```python
from build123d import *

# Parameters (mm, degrees)
SKETCH1_R           = 4.5
SKETCH1_R_2         = 4.15
SKETCH1_R_3         = 1.5
BOSS_EXTRUDE2_DEPTH = 4


with BuildPart() as part:
    # Sketch1 → Boss-Extrude2 (new body)
    with BuildSketch(Plane(origin=(0, 0, 0), x_dir=(1, 0, 0), z_dir=(0, 1, 0))):
        with BuildLine():
            Line((24.492030041, 32), (-16.82364897, 31.38929644))
            ThreePointArc((-16.82364897, 31.38929644), (-26.628373919, 32.520273369), (-35.798432863, 36.170171872))
            Line((-35.798432863, 36.170171872), (-38.479754021, 32.316380416))
            ThreePointArc((-38.479754021, 32.316380416), (-38.105147294, 30.228398184), (-40.193129525, 29.853791457))
            Line((-40.193129525, 29.853791457), (-42.874450683, 26))
            ThreePointArc((-42.874450683, 26), (-33.263093393, 21.189213431), (-22.681899906, 19.302363998))
            Line((-22.681899906, 19.302363998), (24.519122197, 20.000061166))
            ThreePointArc((24.519122197, 20.000061166), (29.912542793, 18.512398384), (34.38564897, 15.151825901))
            ThreePointArc((34.38564897, 15.151825901), (39.572200335, 12.78648108), (44.865586737, 14.901955396))
            ThreePointArc((44.865586737, 14.901955396), (46.941127439, 15.77786367), (49.041095181, 14.962253472))
            ThreePointArc((49.041095181, 14.962253472), (51.498094019, 13.563547988), (54.322847672, 13.445280812))
            ThreePointArc((54.322847672, 13.445280812), (60.067220976, 15.331144894), (65.190877045, 18.540888881))
            ThreePointArc((65.190877045, 18.540888881), (68.785066518, 26.1), (65.156781581, 33.642805002))
            ThreePointArc((65.156781581, 33.642805002), (60.018684596, 36.829381119), (54.265854499, 38.689288065))
            ThreePointArc((54.265854499, 38.689288065), (51.441663661, 38.558267317), (48.991005527, 37.148481859))
            ThreePointArc((48.991005527, 37.148481859), (46.894741967, 36.323397867), (44.815267383, 37.189925399))
            ThreePointArc((44.815267383, 37.189925399), (39.512382816, 39.281476607), (34.336564706, 36.892736755))
            ThreePointArc((34.336564706, 36.892736755), (29.878678322, 33.512000849), (24.492030041, 32))
        make_face()
        with Locations(Location((59.085066518, 26.078100395, 0), (0, 0, 270))):
            Circle(SKETCH1_R, mode=Mode.SUBTRACT)
        with Locations(Location((45.985066518, 26.04852464, 0), (0, 0, 270))):
            Circle(SKETCH1_R_2, mode=Mode.SUBTRACT)
        with Locations(Location((-20.570161775, 25.66516132, 0), (0, 0, 270))):
            Circle(SKETCH1_R_3, mode=Mode.SUBTRACT)
        with BuildLine():
            Line((39.841844345, 34.144341712), (40.83090249, 33.199674393))
            ThreePointArc((40.83090249, 33.199674393), (40.883202658, 30.92140707), (38.604935336, 30.869106902))
            Line((38.604935336, 30.869106902), (37.615877191, 31.813774221))
            ThreePointArc((37.615877191, 31.813774221), (37.563577023, 34.092041544), (39.841844345, 34.144341712))
        make_face(mode=Mode.SUBTRACT)
        with BuildLine():
            Line((52.091670541, 34.171998037), (51.106887992, 33.222874395))
            ThreePointArc((51.106887992, 33.222874395), (51.064875553, 30.944394144), (53.343355804, 30.902381704))
            Line((53.343355804, 30.902381704), (54.328138354, 31.851505346))
            ThreePointArc((54.328138354, 31.851505346), (54.370150793, 34.129985598), (52.091670541, 34.171998037))
        make_face(mode=Mode.SUBTRACT)
        with BuildLine():
            Line((52.128288691, 17.952707568), (51.139230546, 18.897374887))
            ThreePointArc((51.139230546, 18.897374887), (51.086930378, 21.17564221), (53.365197701, 21.227942378))
            Line((53.365197701, 21.227942378), (54.354255846, 20.283275059))
            ThreePointArc((54.354255846, 20.283275059), (54.406556014, 18.005007736), (52.128288691, 17.952707568))
        make_face(mode=Mode.SUBTRACT)
        with BuildLine():
            Line((39.878462495, 17.925051243), (40.863245045, 18.874174885))
            ThreePointArc((40.863245045, 18.874174885), (40.905257484, 21.152655136), (38.626777232, 21.194667576))
            Line((38.626777232, 21.194667576), (37.641994683, 20.245543933))
            ThreePointArc((37.641994683, 20.245543933), (37.599982244, 17.967063682), (39.878462495, 17.925051243))
        make_face(mode=Mode.SUBTRACT)
    extrude(amount=BOSS_EXTRUDE2_DEPTH)


solid = part.part
```
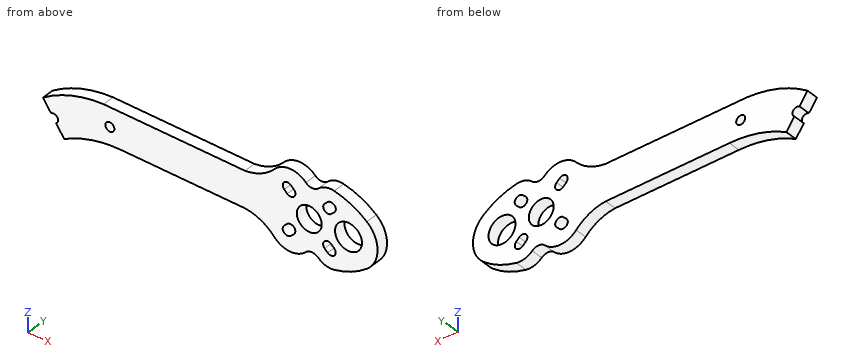
Verification items for the finished model (mm, model axes). Coordinates: 2 decimals unless noted, no trailing zeros. Loops run counter-clockwise (first coordinate to the right, second up) from the corner with the lowest first, then second, coordinate; pieces in that order, holes last. Notation, with made-up numbers: (8.25, 26) - (12.25, 26) arc R18 ccw to (12.25, 41) - close; hole circle Ø4 at (77, 24). An arc over 180 degrees is marked (long way). Put each result on its own line as item: value.
Item 1: Section check D-D (x = -24). Enter the section's corners in (y, z).
Conclusion:
outline: (0, -31.96) - (4, -31.96) - (4, -19.37) - (0, -19.37) - close
Item 2: Gauge pin test, flat end, axial feed: pin 1 Ø5 at (x, z) = (-20.57, -25.67) entering from -Y. Record the tip position at first contact, or that the pin passes through.
Conclusion:
pin 1: stops at y = 0
Item 3: Section check A-A (z = -23). Enter the section's corners in (x, y), then the cut area to 3 significant figures.
Conclusion:
outline: (-37.74, 0) - (43.17, 0) - (43.17, 4) - (-37.74, 4) - close; (48.8, 0) - (55.8, 0) - (55.8, 4) - (48.8, 4) - close; (62.37, 0) - (68.28, 0) - (68.28, 4) - (62.37, 4) - close
area: 375 mm2
Item 4: Scan lines: line 1 along X through (y, z) = (2.75, -18.25); line 2 along X through (y, z) = (3.8, -31); line 3 along X through (y, z) = (0.8, -35). Record each from-to range of solid material in increasing order.
Conclusion:
line 1: x = 30.42 to 37.38, 40.22 to 51.82, 54.6 to 64.82
line 2: x = -37.84 to 38.47, 40.95 to 51.01, 53.44 to 67.44
line 3: x = -36.61 to -33.53, 32.28 to 63.3
Item 5: Section check B-B (x = 28). Enter the section's corners in (y, z), then the cut area to 3 significant figures.
Conclusion:
outline: (0, -32.73) - (4, -32.73) - (4, -19.29) - (0, -19.29) - close
area: 53.8 mm2
Item 6: Section check C-C (y = 2.1). Give the number of separate pieces and of enclosed holes in the cut face, then the cut area to 3 significant figures.
Conclusion:
separate pieces: 1
enclosed holes: 7
area: 1,510 mm2
